```python
from build123d import *
from build123d import SkipClean  # not in build123d's __all__

# Parameters (mm, degrees)
F1_ANGLE = 180
F3_R     = 3
F4_R     = 3
F5_R     = 15


with BuildPart() as f1:
    # F0 (on Front) → F1 (revolve)
    with BuildSketch(Plane.XZ):
        Polygon((15, -18), (23, 0), (3, 120), (0, 120), (0, -25), (18, -25), align=None)
    revolve(axis=Axis((0, 0, 130.329349637), (0, 0, 1)), revolution_arc=F1_ANGLE)

    # F2: F1 across plane


with BuildPart() as f1_1:
    add(f1.part, clean=False)
    with SkipClean():  # cleaning this boolean's faces spoils the solid; the shape is the same uncleaned
        add(f1.part.mirror(Plane.XZ), clean=False)

    # F3
    f3_edges = [f1_1.edges().sort_by_distance(p)[0] for p in [
        (0, 3, 120),
        (0, -3, 120),
    ]]
    fillet(f3_edges, radius=F3_R)

    # F4
    f4_edges = [f1_1.edges().sort_by_distance(p)[0] for p in [
        (0, 15, -18),
        (0, -15, -18),
        (0, 18, -25),
        (0, -18, -25),
    ]]
    fillet(f4_edges, radius=F4_R)

    # F5
    f5_edges = [f1_1.edges().sort_by_distance(p)[0] for p in [
        (0, 23, 0),
        (0, -23, 0),
    ]]
    fillet(f5_edges, radius=F5_R)


solid = f1_1.part
```
Input: part model. Units: mm. Frame: model coordinates. Give positions to 0.01 mm unless a question says otherwise; leave off trailing zeros. Loops run counter-clockwise (first coordinate to the right, second up) from the corner with the lowest first, then second, coordinate; pieces in that order, holes last. Notation, with made-up numbers: M -26.75,11.5 L 12.25,11.5 A35 cw 12.25,43.5 Z; hole C 50.5,37.25 d1. An arc over 180 degrees is marked long. Answer as CSV lines item,"result". Start each with the question number.
1. Section A-A on z = 66. Return loops of the section in (x, y), plus the area to 3 significant figures.
2. Section B-B on z = 94.5. Return loops of the section in (x, y), plus the area to 3 significant figures.
3. Line query: L1, parallel to X at y = -18, z = 12.5; L2, parallel to Y at x = -9.5, z = -15.5; L3, parallel to Y at x = -6.5, z = 55. Output: solid intervals per line, ascending.
4. Pin query (flat end, axial travel): P1, Ø4, axis at x = 3.5, z = 18, coming from the +Y side; P2, Ø5, axis at x = 17, z = 61, coming from the -Y side; P3, Ø10, axis at x = -10, z = 23, coming from the -Y side; P4, Ø2, axis at x = 3.5, z = 60.5, coming from the -Y side. Return the tip coordinate at first contact, or that it passes through.
Computed values:
1,outline,"C 0,0 d24"
1,area,"452 mm²"
2,outline,"C 0,0 d14.5"
2,area,"165 mm²"
3,L1,"x = -10.65 to 10.65"
3,L2,"y = -13.01 to 13.01"
3,L3,"y = -12.21 to 12.21"
4,P1,"stops at y = 20.14"
4,P2,"passes through"
4,P3,"stops at y = -18.74"
4,P4,"stops at y = -12.73"
